The model under review builds one solid part; all positions refer to its coordinate system, in mm. Coordinates: 2 decimals unless noted, no trailing zeros. Order: outer loops, then holes, each group sorted by start corner. A loop starts at its lowest first (then second) coordinate and runs counter-clockwise, first axis right, second up.
```python
from build123d import *

# Parameters (mm, degrees)
F0_R     = 12.7
F2_DEPTH = 152.4
F1_R     = 2.794
F3_DEPTH = 177.8
F4_R     = 2.54
F5_R     = 2.54
F6_DEPTH = 25.4


with BuildPart() as f2:
    # F0 (on Top) → F2 (new body)
    with BuildSketch(Plane.XY):
        Circle(F0_R)
    extrude(amount=F2_DEPTH)

    # F1 (on face) → F3 (cut)
    with BuildSketch(Plane.XY):
        Circle(F1_R)
    extrude(amount=F3_DEPTH, mode=Mode.SUBTRACT)

    # F4
    f4_edges = [f2.edges().sort_by_distance(p)[0] for p in [
        (-12.7, 0, 0),
    ]]
    fillet(f4_edges, radius=F4_R)

    # F5
    f5_edges = [f2.edges().sort_by_distance(p)[0] for p in [
        (-12.7, 0, 152.4),
    ]]
    fillet(f5_edges, radius=F5_R)

    # F6 (cut): a face of the model
    f6_faces = [f2.faces().sort_by_distance(p)[0] for p in [
        (-9.8726318041, 0, 152.4),
    ]]
    extrude(f6_faces, amount=-F6_DEPTH, mode=Mode.SUBTRACT)


solid = f2.part
```
(1) We need section C-C, the plane z = 111.5. Write out the cut boundary in (x, y).
A:
outline: circle Ø25.4 at (0, 0); hole circle Ø5.59 at (0, 0)
(2) Wall thickness on probe 1 along Y at (x, z) = (0, 56); probe 2 along Y at (x, z) = (-0.75, 130); probe 3 along Z at (x, y) = (-1, -7.25): over which ranges is each line inside the solid? List them lowest first.
A:
probe 1: y = -12.7 to -2.79, 2.79 to 12.7
probe 2: y = -12.68 to -10.13, 10.13 to 12.68
probe 3: z = 0 to 127
(3) For pin 1 Ø6 at (x, z) = (4.5, 75.5) entering from -Y; pin 2 Ø3 at (y, z) = (-10, 123) entering from -X; pin 3 Ø10 at (x, y) = (-3.5, -6.5) entering from -Z; pin 4 Ø10 at (x, y) = (-0.5, 1.5) entering from +Z, all flat-tipped, find the tip position at first contact; note any pin that passes through.
A:
pin 1: stops at y = -12.61
pin 2: stops at x = -9.44
pin 3: stops at z = 0
pin 4: stops at z = 127
(4) Draft analysis for pull direction X (two halves, no side actions). For faces 1 (the face through (2.1, -2.1, 127)), 2 (the face through (2.1, -2.1, 0)), 3 (the face through (-2.75, -12.4, 75.17)), 4 (the face through (-2.217, -1.7, 62.611)), state which applies: released by +X, released by -X, zero draft, split by the parting line, or undercut.
A:
face 1: undercut
face 2: zero draft
face 3: split by the parting line
face 4: undercut
(5) We need section A-A, the plane y = 0. Write out the cut boundary in (x, z).
A:
outline: (-12.7, 2.54) arc R2.54 ccw to (-10.16, 0) - (-2.79, 0) - (-2.79, 127) - (-10.16, 127) - (-10.16, 152.4) arc R2.54 ccw to (-12.7, 149.86) - close; (2.79, 0) - (10.16, 0) arc R2.54 ccw to (12.7, 2.54) - (12.7, 149.86) arc R2.54 ccw to (10.16, 152.4) - (10.16, 127) - (2.79, 127) - close
